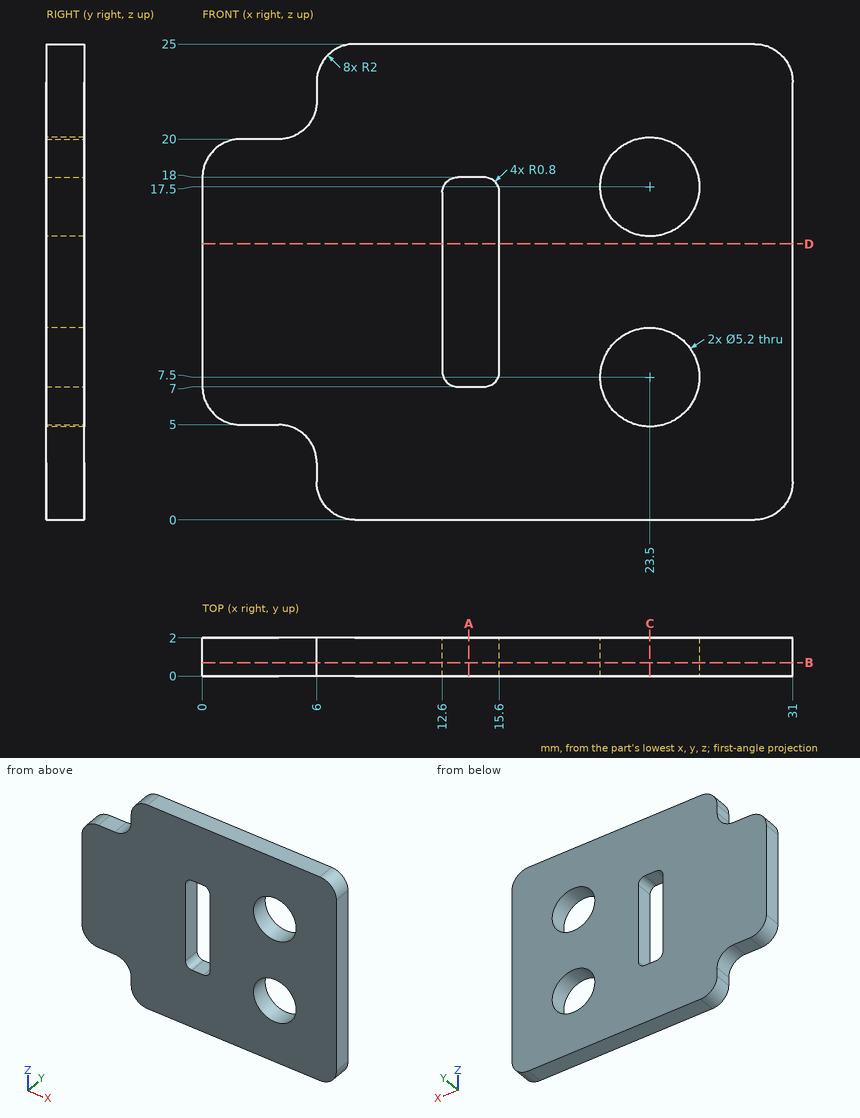
Can you work these out from the drawing? Everything is in mm from the part's minimum corner. Coordinates: 2 decimals unless noted, no trailing zeros. Write each loop counter-clockwise with the first axis right and the second up, starting at its lowest first coordinate (ties: lowest second). Pieces come first, ordered by that corner, then holes. Notation, with made-up numbers: (69.25, 59) - (108.25, 59) arc R21 ccw to (108.25, 68) - close; hole circle Ø5 at (-34, 24.5). An arc over 180 degrees is marked (long way). One line per item, written item: value.
1) I'm going to push flat-ended pins straight in: P1, Ø1.5, axis at x = 16, z = 3.5, coming from the -Y side; P2, Ø1.1, axis at y = 1, z = 22.5, coming from the -X side; P3, Ø4.5, axis at x = 23.5, z = 17.5, coming from the -Y side. Where does each tip first touch, or does it pass through?
Model answer:
P1: stops at y = 0
P2: stops at x = 6
P3: passes through
2) Suppose I cut it at C-C on x = 23.5. Write out the boundary of the cut face in (y, z), and give its area (3 significant figures).
Model answer:
outline: (0, 0) - (2, 0) - (2, 4.9) - (0, 4.9) - close; (0, 10.1) - (2, 10.1) - (2, 14.9) - (0, 14.9) - close; (0, 20.1) - (2, 20.1) - (2, 25) - (0, 25) - close
area: 29.2 mm²
3) Suppose I cut it at B-B on y = 0.7. Write out the boundary of the cut face in (x, z), and give its area (3 significant figures).
Model answer:
outline: (0, 7) arc R2 ccw to (2, 5) - (4, 5) arc R2 cw to (6, 3) - (6, 2) arc R2 ccw to (8, 0) - (29, 0) arc R2 ccw to (31, 2) - (31, 23) arc R2 ccw to (29, 25) - (8, 25) arc R2 ccw to (6, 23) - (6, 22) arc R2 cw to (4, 20) - (2, 20) arc R2 ccw to (0, 18) - close; hole (12.6, 7.8) arc R0.8 ccw to (13.4, 7) - (14.8, 7) arc R0.8 ccw to (15.6, 7.8) - (15.6, 17.2) arc R0.8 ccw to (14.8, 18) - (13.4, 18) arc R0.8 ccw to (12.6, 17.2) - close; hole circle Ø5.2 at (23.5, 7.5); hole circle Ø5.2 at (23.5, 17.5)
area: 637 mm²
4) Suppose I cut it at D-D on z = 14.5. Write out the boundary of the cut face in (x, y), and give its area (3 significant figures).
Model answer:
outline: (0, 0) - (12.6, 0) - (12.6, 2) - (0, 2) - close; (15.6, 0) - (31, 0) - (31, 2) - (15.6, 2) - close
area: 56.0 mm²
5) I need wall thicknesses on line 1 along Z through (x, y) = (23.5, 0.6); line 2 along X through (y, z) = (0.2, 8.5); line 3 along X through (y, z) = (1, 17.75). Which ranges of each line are inside material? Lowest first, please.
Model answer:
line 1: z = 0 to 4.9, 10.1 to 14.9, 20.1 to 25
line 2: x = 0 to 12.6, 15.6 to 21.1, 25.9 to 31
line 3: x = 0 to 12.82, 15.38 to 20.91, 26.09 to 31
6) Suppose I cut it at A-A on x = 14. Write out the boundary of the cut face in (y, z).
Model answer:
outline: (0, 0) - (2, 0) - (2, 7) - (0, 7) - close; (0, 18) - (2, 18) - (2, 25) - (0, 25) - close
